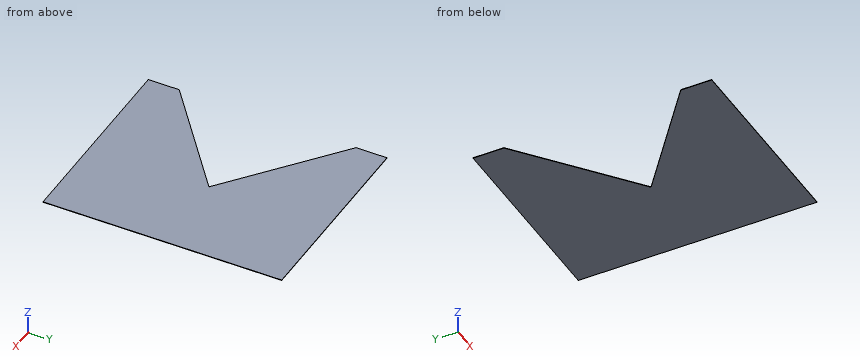
Autodesk Inventor part; units mm, degrees
ref_plane "YZ Plane" through (0, 0, 0) normal (1, 0, 0) x (0, 1, 0)
ref_plane "XZ Plane" through (0, 0, 0) normal (0, 1, 0) x (-1, 0, 0)
ref_plane "XY Plane" through (0, 0, 0) normal (0, 0, 1) x (1, 0, 0)
sketch "Sketch1" plane through (0, 0, 0) normal (0, 0, 1) x (1, 0, 0)
  line L0 (0, -810) -> (1345, -810)
  line L1 (1345, -810) -> (1345, 810)
  line L2 (1345, 810) -> (0, 810)
  line L3 (0, 810) -> (0, -810)
  point P0 (0, 0)
  point P1 (0, 0)
  dimension "d0" = 1345
  dimension "d1" = 1620
extrude "Plate1" add sketch "Sketch1" along normal blind 3
sketch "Sketch5" plane through (0, 0, 0) normal (0, 0, -1) x (-1, 0, 0)
  line L0 (0, -810) -> (-1345, -810) construction
  line L1 (0, 810) -> (0, -810)
  line L2 (-1345, 810) -> (0, 810) construction
  line L3 (-1345, -810) -> (-1345, 810) construction
  line L4 (0, -600) -> (-750, 0)
  line L5 (-750, 0) -> (0, 600)
  line L6 (12.3081, -1975.0573) -> (-487.6919, -1975.0573)
  line L7 (-487.6919, -1975.0573) -> (-487.6919, -2425.2593)
  line L8 (-487.6919, -2425.2593) -> (12.3081, -1975.0573)
  point P0 (0, 0)
  point P1 (0, 0)
  dimension "d26" = 500
  dimension "d27" = 48
  dimension "d28" = 672.8164
  dimension "d29" = 750
  dimension "d30" = 1200
extrude "Cut1" cut sketch "Sketch5" against normal blind 3 contours L1 L4 L5
equation "\"d31\" = Thickness"
equation "\"d2\" = Thickness"
equation "\"BendReliefWidth\" = Thickness"
equation "\"BendReliefDepth\" = 0.5 * Thickness"
equation "\"CornerReliefSize\" = 4 * Thickness"
equation "\"MinimumRemnant\" = 2 * Thickness"
equation "\"TransitionRadius\" = BendRadius"
equation "\"JacobiRadiusSize\" = BendRadius"
equation "\"GapSize\" = Thickness"
properties part number "BSH 014 board cone 4" material "09g2s"
Input: part model. Units: mm. Frame: model coordinates. Coordinates: 2 decimals unless noted, no trailing zeros. Write each loop counter-clockwise with the first axis right and the second up, starting at its lowest first coordinate (ties: lowest second). Pieces come first, ordered by that corner, then holes. Notation, with made-up numbers: (69.25, 10) -> (110.25, 10) arc R19 ccw to (110.25, 25) -> close; hole circle Ø11 at (-32, 25). An arc over 180 degrees is marked (long way). Write each question's results on one line, items separated by ' | '.
Item 1: Section query D-D on x = 688.5. Return loops of the section in (y, z), plus the area to 3 significant figures.
Conclusion:
outline: (-810, 0) -> (-49.2, 0) -> (-49.2, 3) -> (-810, 3) -> close; (49.2, 0) -> (810, 0) -> (810, 3) -> (49.2, 3) -> close | area: 4,560 mm^2
Item 2: Section query C-C on y = -317. Return loops of the section in (x, z), plus the area to 3 significant figures.
Conclusion:
outline: (353.75, 0) -> (1345, 0) -> (1345, 3) -> (353.75, 3) -> close | area: 2,970 mm^2
Item 3: Section query A-A on x = 451.5. Return loops of the section in (y, z).
Conclusion:
outline: (-810, 0) -> (-238.8, 0) -> (-238.8, 3) -> (-810, 3) -> close; (238.8, 0) -> (810, 0) -> (810, 3) -> (238.8, 3) -> close
Item 4: Section query B-B on z = 0.9. Return loops of the section in (x, y).
Conclusion:
outline: (0, -810) -> (1345, -810) -> (1345, 810) -> (0, 810) -> (0, 600) -> (750, 0) -> (0, -600) -> close
Item 5: Material intervals for probe 1 along Y at (x, z) = (225.5, 2.6); probe 2 along Y at (x, z) = (613.5, 1.3); probe 3 along X at (y, z) = (-33.5, 2.1) (3 decimals), sorted ascending.
Conclusion:
probe 1: y = -810 to -419.6, 419.6 to 810 | probe 2: y = -810 to -109.2, 109.2 to 810 | probe 3: x = 708.125 to 1345
